```python
from build123d import *

# Parameters (mm, degrees)
SKETCH2_W           = 75
SKETCH2_H           = 13.5
SKETCH2_R           = 2
BOSS_EXTRUDE1_DEPTH = 13.5
CUT_EXTRUDE1_DEPTH  = 13.5


with BuildPart() as part:
    # Sketch2 → Boss-Extrude1 (new body)
    with BuildSketch(Plane.XY):
        with Locations((37.5, 6.75)):
            Rectangle(SKETCH2_W, SKETCH2_H)
        with Locations((6, 6.75)):
            Circle(SKETCH2_R, mode=Mode.SUBTRACT)
        with Locations((14, 6.75)):
            Circle(SKETCH2_R, mode=Mode.SUBTRACT)
        with Locations((69, 6.75)):
            Circle(SKETCH2_R, mode=Mode.SUBTRACT)
        with Locations((61, 6.75)):
            Circle(SKETCH2_R, mode=Mode.SUBTRACT)
    extrude(amount=BOSS_EXTRUDE1_DEPTH)

    # Sketch3 → Cut-Extrude1 (cut)
    with BuildSketch(Plane(origin=(0, 13.5, 0), x_dir=(1, 0, 0), z_dir=(0, 1, 0))):
        with BuildLine():
            ThreePointArc((37.5, -3.349632373), (28.25, -6.75), (37.5, -10.150367627))
            ThreePointArc((37.5, -10.150367627), (46.75, -6.75), (37.5, -3.349632373))
        make_face()
    extrude(amount=-CUT_EXTRUDE1_DEPTH, mode=Mode.SUBTRACT)


solid = part.part
```
Part model, mm, in its own coordinate system. Coordinates: 2 decimals unless noted, no trailing zeros. Order: outer loops, then holes, each group sorted by start corner. A loop starts at its lowest first (then second) coordinate and runs counter-clockwise, first axis right, second up. Notation, with made-up numbers: (38, -3.75) - (67, -3.75) arc R29 cw to (67, 26.25) - close; hole circle Ø1 at (-8, 38.25). An arc over 180 degrees is marked (long way). Return JSON: item names as keys, results as strings. Group by question number.
Item 1: Pull direction Z, two halves, no side cores. Call faces 1 (the face through (28.253, 6.844, 6.571)), 2 (the face through (37, 7, 13.5)), 3 (the face through (0, 7, 7)): pulls with the +Z half, pulls with the -Z half, needs draft (parallel to the pull), parting line crosses it, or undercut.
Item 2: Cut at C-C (z = 2.5). List the corners of the cut face in (x, y).
Item 3: Cut at A-A (z = 6.75). List the corners of the cut face in (x, y), plus the area to 3 significant figures.
Item 4: Cut at D-D (y = 8). List the corners of the cut face in (x, z), plus the area to 3 significant figures.
Item 5: Cut at B-B (x = 14). List the corners of the cut face in (y, z), plus the area to 3 significant figures.
Item 6: Drill centre lines: probe 1 along Z at (x, y) = (33.5, 3.5); probe 2 along Y at (x, z) = (61, 7.5); probe 3 along X at (y, z) = (8.25, 1.25). Where is each one in solid material? Low to high. Write a range as from..to.
Check values:
{
 "1": {"face 1": "undercut", "face 2": "pulls with the +Z half", "face 3": "needs draft"},
 "2": {"outline": "(0, 0) - (30.42, 0) - (30.42, 13.5) - (0, 13.5) - close; (36.58, 0) - (38.42, 0) - (38.42, 13.5) - (36.58, 13.5) - close; (44.58, 0) - (75, 0) - (75, 13.5) - (44.58, 13.5) - close; hole circle Ø4 at (6, 6.75); hole circle Ø4 at (14, 6.75); hole circle Ø4 at (61, 6.75); hole circle Ø4 at (69, 6.75)"},
 "3": {"outline": "(0, 0) - (28.25, 0) - (28.25, 13.5) - (0, 13.5) - close; (46.75, 0) - (75, 0) - (75, 13.5) - (46.75, 13.5) - close; hole circle Ø4 at (6, 6.75); hole circle Ø4 at (14, 6.75); hole circle Ø4 at (61, 6.75); hole circle Ø4 at (69, 6.75)", "area": "712 mm2"},
 "4": {"outline": "(0, 0) - (4.44, 0) - (4.44, 13.5) - (0, 13.5) - close; (7.56, 0) - (12.44, 0) - (12.44, 13.5) - (7.56, 13.5) - close; (15.56, 0) - (59.44, 0) - (59.44, 13.5) - (15.56, 13.5) - close; (62.56, 0) - (67.44, 0) - (67.44, 13.5) - (62.56, 13.5) - close; (70.56, 0) - (75, 0) - (75, 13.5) - (70.56, 13.5) - close; hole (37.5, 3.35) arc R5.25 ccw (long way) to (37.5, 10.15) arc R5.25 ccw (long way) to start", "area": "682 mm2"},
 "5": {"outline": "(0, 0) - (4.75, 0) - (4.75, 13.5) - (0, 13.5) - close; (8.75, 0) - (13.5, 0) - (13.5, 13.5) - (8.75, 13.5) - close", "area": "128 mm2"},
 "6": {"probe 1": "z = 0..1.5, 12..13.5", "probe 2": "y = 0..4.75, 8.75..13.5", "probe 3": "x = 0..4.68, 7.32..12.68, 15.32..59.68, 62.32..67.68, 70.32..75"}
}
